For this review, take the finished solid that the model builds, in its own axes (mm). Round coordinates to 2 decimals unless told otherwise and drop trailing zeros. Write each loop counter-clockwise with the first axis right and the second up, starting at its lowest first coordinate (ties: lowest second). Pieces come first, ordered by that corner, then holes. Notation, with made-up numbers: M 4,37 L 11,37 A30 cw 11,68 Z; hole C 36,85.5 d11. An arc over 180 degrees is marked long. Write each question's results on one line, items separated by ' | '. Start each with the question number.
Autodesk Inventor part; units mm, degrees
ref_plane "YZ Plane" through (0, 0, 0) normal (1, 0, 0) x (0, 1, 0)
ref_plane "XZ Plane" through (0, 0, 0) normal (0, 1, 0) x (-1, 0, 0)
ref_plane "XY Plane" through (0, 0, 0) normal (0, 0, 1) x (1, 0, 0)
sketch "Sketch1" plane through (0, 0, 0) normal (0, 1, 0) x (-1, 0, 0)
  line L0 (-20, 40) -> (20, 40)
  line L1 (20, 40) -> (20, -40)
  line L2 (20, -40) -> (-20, -40)
  line L3 (-20, -40) -> (-20, 40)
  line L4 (-20, 40) -> (20, -40) construction
  line L5 (20, 40) -> (-20, -40) construction
  line L6 (-17.76, 37.76) -> (17.76, 37.76)
  line L7 (17.76, 37.76) -> (17.76, -37.76)
  line L8 (17.76, -37.76) -> (-17.76, -37.76)
  line L9 (-17.76, -37.76) -> (-17.76, 37.76)
  line L10 (-17.76, 37.76) -> (17.76, -37.76) construction
  line L11 (17.76, 37.76) -> (-17.76, -37.76) construction
  point P0 (0, 0)
  dimension "d0" = 40
  dimension "d1" = 80
  dimension "d2" = 35.52
  dimension "d10" = 2.24
extrude "Extrusion1" add sketch "Sketch1" along normal blind 1824.7
fillet "Fillet1" radius 2 4 edges at (-17.76, 912.35, 37.76) (17.76, 912.35, -37.76) (17.76, 912.35, 37.76) (-17.76, 912.35, -37.76)
fillet "Fillet1" radius 4 4 edges at (20, 912.35, 40) (-20, 912.35, 40) (20, 912.35, -40) (-20, 912.35, -40)
sketch "Boceto3" plane through (-16, 0, 40) normal (0, 0, 1) x (1, 0, 0)
  circle A0 centre (16, 11.25) radius 4.5
  circle A1 centre (16, 68.75) radius 4.5
  circle A2 centre (16, 911.25) radius 4.5
  circle A3 centre (16, 968.75) radius 4.5
  circle A4 centre (16, 1268.75) radius 4.5
  circle A5 centre (16, 1211.25) radius 4.5
  circle A6 centre (16, 968.75) radius 5.5
  circle A7 centre (16, 911.25) radius 5.5
  circle A8 centre (16, 68.75) radius 5.5
  circle A9 centre (16, 11.25) radius 5.5
  circle A10 centre (16, 1268.75) radius 5.5
  circle A11 centre (16, 1211.25) radius 5.5
  point P0 (16, 0)
  dimension "d11" = 11
  dimension "d12" = 11
  dimension "d13" = 11
  dimension "d14" = 11
  dimension "d15" = 11
  dimension "d16" = 11
extrude "Extrusión3" cut sketch "Boceto3" against normal blind 10 contours A0 | A1 | A2 | A3 | A4 | A5 | A6 | A7 | A8 | A9 | A10 | A11
sketch "Sketch8" plane through (20, 0, 36) normal (1, 0, 0) x (0, 0, -1)
  circle A0 centre (47.8764, 1770.0887) radius 11.11
  point P0 (36, 0)
extrude "Extrusion7" cut sketch "Sketch8" against normal through all
properties part number "tubo2-40x40x1800" material "Acero, carbono"
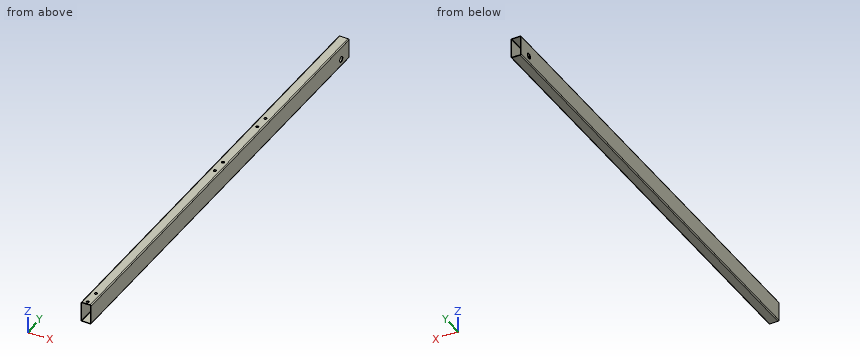
Item 1: We need section B-B on z = 21. State the section outline as (x, y) points.
Item 2: Insertion check: P1, Ø20, axis at y = 1770.09, z = -11.88, coming from the +X side. The pin has a flat end and moves straight along its axis. Give the tip position at first contact, or say it passes through.
Item 3: We need section A-A on y = 167. State the section outline as (x, z) points, then the cut area to 3 significant figures.
Item 4: For probe 1 along Z at (x, y) = (-7.5, 470); probe 2 along X at (y, z) = (1029, 25.5); probe 3 along X at (y, z) = (642, 36.5), list the stretches that pass through material, from the lowest coordinate up.
Numbers:
1) outline: M -20,0 L -17.76,0 L -17.76,1824.7 L -20,1824.7 Z; M 17.76,0 L 20,0 L 20,1824.7 L 17.76,1824.7 Z
2) P1: passes through
3) outline: M -20,-36 A4 ccw -16,-40 L 16,-40 A4 ccw 20,-36 L 20,36 A4 ccw 16,40 L -16,40 A4 ccw -20,36 Z; hole M -17.76,-35.76 A2 ccw -15.76,-37.76 L 15.76,-37.76 A2 ccw 17.76,-35.76 L 17.76,35.76 A2 ccw 15.76,37.76 L -15.76,37.76 A2 ccw -17.76,35.76 Z | area: 507 mm^2
4) probe 1: z = -40 to -37.76, 37.76 to 40 | probe 2: x = -20 to -17.76, 17.76 to 20 | probe 3: x = -19.97 to -17.62, 17.62 to 19.97
